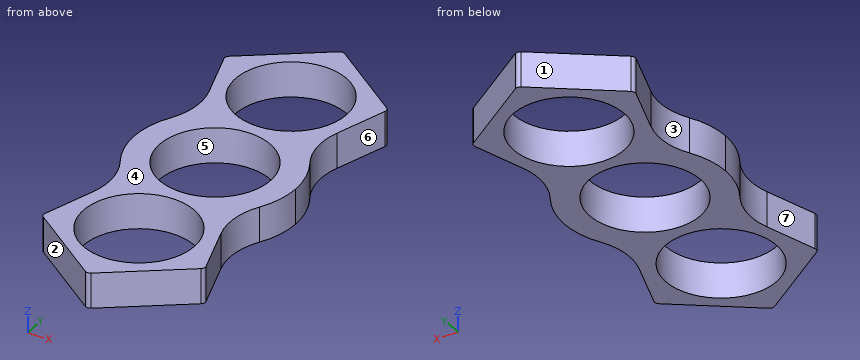
from build123d import *
from build123d import SkipClean  # not in build123d's __all__

# Parameters (mm, degrees)
F1_DEPTH = 3.5
F3_R     = 11
F4_DEPTH = 7.001


with BuildPart() as f1:
    # F0 (on Top) → F1 (new body, symmetric)
    with BuildSketch(Plane.XY):
        with BuildLine():
            ThreePointArc((-11, 0), (0, 11), (11, 0))
            Line((11, 0), (16, 0))
            ThreePointArc((16, 0), (15.4421025537, 4.1882536601), (13.8073164099, 8.0844303175))
            ThreePointArc((13.8073164099, 8.0844303175), (12.1011838507, 13.2547074929), (12.6620262811, 18.6702508773))
            Line((12.6620262811, 18.6702508773), (15.9510565163, 28.7928450855))
            ThreePointArc((15.9510565163, 28.7928450855), (15.9510565163, 29.4108790743), (15.5877852523, 29.9108790743))
            Line((15.5877852523, 29.9108790743), (0.5877852523, 40.8090169944))
            ThreePointArc((0.5877852523, 40.8090169944), (0, 41), (-0.5877852523, 40.8090169944))
            Line((-0.5877852523, 40.8090169944), (-15.5877852523, 29.9108790743))
            ThreePointArc((-15.5877852523, 29.9108790743), (-15.9510565163, 29.4108790743), (-15.9510565163, 28.7928450855))
            Line((-15.9510565163, 28.7928450855), (-12.6620262811, 18.6702508773))
            ThreePointArc((-12.6620262811, 18.6702508773), (-12.1011838507, 13.2547074929), (-13.8073164099, 8.0844303175))
            ThreePointArc((-13.8073164099, 8.0844303175), (-15.4421025537, 4.1882536601), (-16, 0))
            Line((-16, 0), (-11, 0))
        make_face()
    extrude(amount=F1_DEPTH, both=True)

    # F2: F1 across face


with BuildPart() as f1_1:
    add(f1.part, clean=False)
    with SkipClean():  # cleaning this boolean's faces spoils the solid; the shape is the same uncleaned
        add(f1.part.mirror(Plane(origin=(-13.5, 0, 0), x_dir=(1, 0, 0), z_dir=(0, -1, 0))), clean=False)

    # F3 (on face) → F4 (cut, through all)
    with BuildSketch(Plane.XY.offset(3.5)):
        with Locations((0, 24.5)):
            Circle(F3_R)
        with Locations((0, -24.5)):
            Circle(F3_R)
    extrude(amount=-F4_DEPTH, mode=Mode.SUBTRACT)


solid = f1_1.part
For this review, take the finished solid that the model builds, in its own axes (mm). Face numbers are marked on the shaded views. A direction names the side the tool comes from. Round coordinates to 2 decimals unless told otherwise and drop trailing zeros. Write each loop counter-clockwise with the first axis right and the second up, starting at its lowest first coordinate (ties: lowest second). Pieces come first, ordered by that corner, then holes. Notation, with made-up numbers: (67, 24.25) -> (76, 24.25) arc R24 ccw to (76, 62.25) -> close; hole circle Ø7 at (78, 3). An arc over 180 degrees is marked (long way). Use CSV: the item, a comma, the result in double quotes.
(1) Consider section D-D, the plane x = -4.5. Give the boundary of the cut face in (y, z), plus the area to 3 significant figures.
Computed values:
outline,"(-37.97, -3.5) -> (-34.54, -3.5) -> (-34.54, 3.5) -> (-37.97, 3.5) -> close; (-14.46, -3.5) -> (-10.04, -3.5) -> (-10.04, 3.5) -> (-14.46, 3.5) -> close; (10.04, -3.5) -> (14.46, -3.5) -> (14.46, 3.5) -> (10.04, 3.5) -> close; (34.54, -3.5) -> (37.97, -3.5) -> (37.97, 3.5) -> (34.54, 3.5) -> close"
area,"110 mm²"
(2) Clearance check with flat-ended pins moving along their axes: P1, Ø2, axis at y = -16.5, z = -2, coming from the +X side; P2, Ø1.5, axis at y = 23.5, z = 0, coming from the -X side (3 decimals); P3, Ø1, axis at y = -30.5, z = 2.5, coming from the +X side. State where each tip first meets the part, or that it passes through.
Computed values:
P1,"x = 12.34"
P2,"x = -14.475"
P3,"x = 15.47"
(3) For the marked faces 5, 6 and 7, list the 3-axis set-ups (+Z, -Z, +X, -X, +Y, -Y) from which the entire face can be reached by the end or side of a thin tool; tool diameter is ignored.
Computed values:
face 5,"+Z, -Z"
face 6,"+Z, -Z, +X"
face 7,"+Z, -Z, -X"
(4) Consider section B-B, the plane y = 15.5. Give the boundary of the cut face in (x, z).
Computed values:
outline,"(-12.05, -3.5) -> (-6.32, -3.5) -> (-6.32, 3.5) -> (-12.05, 3.5) -> close; (6.32, -3.5) -> (12.05, -3.5) -> (12.05, 3.5) -> (6.32, 3.5) -> close"
(5) Consider section C-C, the plane x = -9. Give the boundary of the cut face in (y, z).
Computed values:
outline,"(-34.7, -3.5) -> (-30.82, -3.5) -> (-30.82, 3.5) -> (-34.7, 3.5) -> close; (-18.18, -3.5) -> (-6.32, -3.5) -> (-6.32, 3.5) -> (-18.18, 3.5) -> close; (6.32, -3.5) -> (18.18, -3.5) -> (18.18, 3.5) -> (6.32, 3.5) -> close; (30.82, -3.5) -> (34.7, -3.5) -> (34.7, 3.5) -> (30.82, 3.5) -> close"
(6) Consider section A-A, the plane z = 1.25. Give the boundary of the cut face in (x, y), plus the area to 3 significant figures.
Computed values:
outline,"(-15.95, -28.79) arc R1 ccw to (-15.59, -29.91) -> (-0.59, -40.81) arc R1 ccw to (0.59, -40.81) -> (15.59, -29.91) arc R1 ccw to (15.95, -28.79) -> (12.66, -18.67) arc R13 cw to (13.81, -8.08) arc R16 ccw to (13.81, 8.08) arc R13 cw to (12.66, 18.67) -> (15.95, 28.79) arc R1 ccw to (15.59, 29.91) -> (0.59, 40.81) arc R1 ccw to (-0.59, 40.81) -> (-15.59, 29.91) arc R1 ccw to (-15.95, 28.79) -> (-12.66, 18.67) arc R13 cw to (-13.81, 8.08) arc R16 ccw to (-13.81, -8.08) arc R13 cw to (-12.66, -18.67) -> close; hole circle Ø22 at (0, -24.5); hole circle Ø22 at (0, 0); hole circle Ø22 at (0, 24.5)"
area,"885 mm²"
(7) Draft analysis for pull direction Y (two halves, no side actions). For the marked faces 1, 2, 3 and 4, state which applies: +Y half, -Y half, draft (parallel to the pull), parting line (faces both ways), or undercut.
Computed values:
face 1,"+Y half"
face 2,"-Y half"
face 3,"undercut"
face 4,"draft"
(8) To check wall thickness, follow L1, parallel to Y at x = 5, z = -3; L2, parallel to Y at x = 10, z = 0; L3, parallel to X at y = 0, z = -0.5. State the ranges of each line that lie inside material, in increasing order. Write a range as [from, to].
Computed values:
L1,"[-37.6, -34.3], [-14.7, -9.8], [9.8, 14.7], [34.3, 37.6]"
L2,"[-33.97, -29.08], [-19.92, -4.58], [4.58, 19.92], [29.08, 33.97]"
L3,"[-16, -11], [11, 16]"
